Autodesk Inventor part; units mm, degrees
ref_plane "YZ Plane" through (0, 0, 0) normal (1, 0, 0) x (0, 1, 0)
ref_plane "XZ Plane" through (0, 0, 0) normal (0, 1, 0) x (-1, 0, 0)
ref_plane "XY Plane" through (0, 0, 0) normal (0, 0, 1) x (1, 0, 0)
sketch "Boceto1" plane through (0, 0, 0) normal (0, 1, 0) x (-1, 0, 0)
  line L0 (53, 63) -> (-53, 63)
  line L1 (-53, 63) -> (-53, -63)
  line L2 (-53, -63) -> (53, -63)
  line L3 (53, -63) -> (53, 63)
  point P0 (0, 0)
  point P1 (0, 63)
  dimension "d1" = 106
  dimension "d2" = 126
  dimension "d3" = 53
  dimension "d4" = 63
extrude "Extrusión1" add sketch "Boceto1" along normal blind 5
sketch "Boceto2" plane through (0, 5, 0) normal (0, 1, 0) x (1, 0, 0)
  circle A0 centre (-45.929, -42.384) radius 1.5
  line L0 (-53, -63) -> (53, -63)
  line L1 (-53, 63) -> (-53, -63)
  line L2 (-81, 0) -> (77, 0)
  line L3 (0, -130) -> (0, 128)
  circle A1 centre (-45.929, 42.384) radius 1.5
  line L4 (-53, -63) -> (-53, 63)
  circle A2 centre (45.929, -42.384) radius 1.5
  circle A3 centre (45.929, 42.384) radius 1.5
  point P0 (0, 0)
  dimension "d7" = 3
  dimension "d8" = 20.616
  dimension "d9" = 7.071
extrude "Extrusión2" add sketch "Boceto2" along normal blind 10 contours A0 | A1 | A2 | A3
sketch "Boceto3" plane through (0, 0, 0) normal (0, -1, 0) x (1, 0, 0)
  line L0 (-35, 52.5) -> (35, 52.5)
  line L1 (35, 52.5) -> (35, -52.5)
  line L2 (35, -52.5) -> (-35, -52.5)
  line L3 (-35, -52.5) -> (-35, 52.5)
  line L4 (53, -63) -> (-53, -63)
  line L5 (-53, 63) -> (53, 63)
  line L6 (53, 63) -> (53, -63)
  line L7 (-53, -63) -> (-53, 63)
  line L8 (35, 17.5) -> (-35, 17.5)
  line L9 (35, -17.5) -> (-35, -17.5)
  line L10 (0, 52.5) -> (0, -52.5)
  point P0 (0, 0)
  point P1 (0, 17.5)
  point P2 (0, -17.5)
  dimension "d12" = 52.5
  dimension "d13" = 126
  dimension "d14" = 106
  dimension "d15" = 52.5
  dimension "d16" = 35
  dimension "d17" = 35
  dimension "d18" = 35
  dimension "d19" = 35
  dimension "d20" = 35
extrude "Extrusión3" cut sketch "Boceto3" against normal blind 2 contours L0 L10 L8 L3 | L0 L1 L8 L10 | L8 L1 L9 L10
properties part number "Tapa 0"
Could you check a few things on this model? Use its own coordinates, in mm. A direction names the side the tool comes from. Give positions to 0.01 mm unless a question says otherwise; leave off trailing zeros. Loops run counter-clockwise (first coordinate to the right, second up) from the corner with the lowest first, then second, coordinate; pieces in that order, holes last. Notation, with made-up numbers: (-29, -30) -> (22, -30) arc R12 cw to (22, -7) -> close; hole circle Ø3 at (-17, 32.25). An arc over 180 degrees is marked (long way). Return JSON: item names as keys, results as strings.
Item 1: I need wall thicknesses on L1, parallel to Z at x = 23.5, y = 1.5; L2, parallel to X at y = 0.75, z = 44; L3, parallel to X at y = 1, z = -11.5. Which ranges of each line are inside material? Lowest first, please. Write a range as from..to.
Geometry results:
{"L1": "z = -63..-17.5, 52.5..63", "L2": "x = -53..-35, 35..53", "L3": "x = -53..0, 35..53"}
Item 2: If we section it at A-A on x = 13: List the corners of the cut face in (y, z) for me, plus the area to 3 significant figures.
Geometry results:
{"outline": "(0, -63) -> (5, -63) -> (5, 63) -> (0, 63) -> (0, 52.5) -> (2, 52.5) -> (2, -17.5) -> (0, -17.5) -> close", "area": "490 mm²"}
Item 3: Which directions (+Z, -Z, +X, -X, +Y, -Y) give clear straight access to the entire face, cutting with the end or side of a thin tool? Please do faces 5 (the cylindrical face through (-47.12, 9.93, 41.47)), 6 (the flat face through (1, 2, -63)).
Geometry results:
{"face 5": "+Y", "face 6": "-Z, +X, -X, +Y, -Y"}
Item 4: If we section it at C-C on y = 6.5: List the corners of the cut face in (x, z) for me, plus the area to 3 significant figures.
Geometry results:
{"outline": "circle Ø3 at (-45.93, -42.38); circle Ø3 at (-45.93, 42.38); circle Ø3 at (45.93, -42.38); circle Ø3 at (45.93, 42.38)", "area": "28.3 mm²"}
Item 5: We'd pull the mould along X, two halves only. Please class faces 1 (the flat face through (-1, 2, 63)), 2 (the flat face through (53, 2, 1)), 3 (the flat face through (7, 2, 26)), 4 (the cylindrical face through (46.621, 9.93, -43.715)): +X half, -X half, draft (parallel to the pull), parting line (faces both ways), or undercut.
Geometry results:
{"face 1": "draft", "face 2": "+X half", "face 3": "undercut", "face 4": "undercut"}
Item 6: If we section it at B-B on z = 4: List the corners of the cut face in (x, y) for me, plus the area to 3 significant figures.
Geometry results:
{"outline": "(-53, 0) -> (0, 0) -> (0, 2) -> (35, 2) -> (35, 0) -> (53, 0) -> (53, 5) -> (-53, 5) -> close", "area": "460 mm²"}
Item 7: I'm going to push flat-ended pins straight in: pin 1 (5 mm diameter, centred on x = 28.5, z = -17, fed in from +Y); pin 2 (8 mm diameter, centred on x = -28, y = 5.5, fed in from -Z); pin 3 (1.5 mm diameter, centred on x = 29.5, z = 46.5, fed in from -Y). Where does each tip first touch, or does it pass through?
Geometry results:
{"pin 1": "stops at y = 5", "pin 2": "stops at z = -63", "pin 3": "stops at y = 2"}
Item 8: If we section it at D-D on z = -50: List the corners of the cut face in (x, y) for me, plus the area to 3 significant figures.
Geometry results:
{"outline": "(-53, 0) -> (53, 0) -> (53, 5) -> (-53, 5) -> close", "area": "530 mm²"}
